from build123d import *

# Parameters (mm, degrees)
F0_W      = 133.35
F0_H      = 57.15
F0_W_2    = 94.615
F0_H_2    = 4.064
F0_W_3    = 10.16
F0_H_3    = 42.545
F1_DEPTH  = 3.81
F2_W      = 5.6896
F2_H      = 39.37
F3_DEPTH  = 31.75
F4_R      = 5.08
F5_R      = 10.287
F6_DEPTH  = 25.4
F7_R      = 2.0701
F8_DEPTH  = 3.811
F9_R      = 5.08
F10_R     = 1.27
F11_R     = 12.7
F11_R_2   = 10.287
F12_DEPTH = 4.6736
F13_DEPTH = 15.494
F14_R     = 2.54
F15_DEPTH = 5.08
F16_R     = 2.54
F17_DEPTH = 25.4
F18_R     = 2.54
F19_DEPTH = 25.4
F20_R     = 2.54
F21_DEPTH = 25.4
F22_R     = 5.07999


# Not quite as in the source:
# - a fillet or chamfer is up to 0.001 mm smaller than in the source, because OpenCascade refuses the exact size


with BuildPart() as f1:
    # F0 (on Top) → F1 (new body)
    with BuildSketch(Plane.XY):
        Rectangle(F0_W, F0_H)
        Polygon((57.4675, -21.2725), (57.4675, -25.3365), (47.3075, -25.3365), (-47.3075, -25.3365), (-57.4675, -25.3365), (-57.4675, -21.2725), (-57.4675, 21.2725), (-57.4675, 25.3365), (-47.3075, 25.3365), (47.3075, 25.3365), (57.4675, 25.3365), (57.4675, 21.2725), align=None, mode=Mode.SUBTRACT)
        with Locations((0, 23.3045)):
            Rectangle(F0_W_2, F0_H_2)
        with Locations((-52.3875, 0)):
            Rectangle(F0_W_3, F0_H_3)
        with Locations((-52.3875, -23.3045)):
            Rectangle(F0_W_3, F0_H_2)
        with Locations((0, -23.3045)):
            Rectangle(F0_W_2, F0_H_2)
        Rectangle(F0_W_2, F0_H_3)
        with Locations((52.3875, 0)):
            Rectangle(F0_W_3, F0_H_3)
        with Locations((52.3875, -23.3045)):
            Rectangle(F0_W_3, F0_H_2)
        with Locations((52.3875, 23.3045)):
            Rectangle(F0_W_3, F0_H_2)
        with Locations((-52.3875, 23.3045)):
            Rectangle(F0_W_3, F0_H_2)
    extrude(amount=F1_DEPTH)

    # F2 (on face) → F3 (join)
    with BuildSketch(Plane.XY.offset(3.81)):
        with Locations((-63.8302, 0.0610498762)):
            Rectangle(F2_W, F2_H)
    extrude(amount=F3_DEPTH)

    # F4
    f4_edges = [f1.edges().sort_by_distance(p)[0] for p in [
        (-63.8302, 19.74605, 35.56),
        (-63.8302, -19.62395, 35.56),
    ]]
    fillet(f4_edges, radius=F4_R)

    # F5 (on face) → F6 (cut)
    with BuildSketch(Plane(origin=(-66.675, 0, 0), x_dir=(0, -1, 0), z_dir=(-1, 0, 0))):
        with Locations((0, 17.145)):
            Circle(F5_R)
    extrude(amount=-F6_DEPTH, mode=Mode.SUBTRACT)

    # F7 (on face) → F8 (cut, through all)
    with BuildSketch(Plane.XY.offset(3.81)):
        with Locations((-62.5474974513, 24.164236586)):
            Circle(F7_R)
        with Locations((62.3570047319, 24.7649991388)):
            Circle(F7_R)
        with BuildLine():
            ThreePointArc((64.4271047319, -24.7650008612), (64.1570098525, -23.7426038856), (63.4172061032, -22.987))
            Line((63.4172061032, -22.987), (61.2968033606, -22.987))
            ThreePointArc((61.2968033606, -22.987), (61.3346077563, -26.5650059818), (64.4271047319, -24.7650008612))
        make_face()
        with BuildLine():
            Line((61.2968033606, -22.987), (63.4172061032, -22.987))
            ThreePointArc((63.4172061032, -22.987), (62.3570047319, -22.6949008612), (61.2968033606, -22.987))
        make_face()
        with Locations((-62.5474974513, -24.7649997473)):
            Circle(F7_R)
    extrude(amount=-F8_DEPTH, mode=Mode.SUBTRACT)

    # F9
    f9_edges = [f1.edges().sort_by_distance(p)[0] for p in [
        (66.675, 28.575, 1.905),
        (-66.675, 28.575, 1.905),
        (-66.675, -28.575, 1.905),
        (66.675, -28.575, 1.905),
    ]]
    fillet(f9_edges, radius=F9_R)

    # F10
    f10_edges = [f1.edges().sort_by_distance(p)[0] for p in [
        (-66.675, 0.06105, 35.56),
    ]]
    fillet(f10_edges, radius=F10_R)

    # F11 (on face) → F12 (cut)
    with BuildSketch(Plane.YZ.offset(-60.9854)):
        with Locations((0, 17.145)):
            Circle(F11_R)
        with Locations((0, 17.145)):
            Circle(F11_R_2, mode=Mode.SUBTRACT)
    extrude(amount=-F12_DEPTH, mode=Mode.SUBTRACT)

    # F0 (on Top) → F13 (join)
    with BuildSketch(Plane.XY):
        with Locations((52.3875, 23.3045)):
            Rectangle(F0_W_3, F0_H_2)
        with Locations((52.3875, -23.3045)):
            Rectangle(F0_W_3, F0_H_2)
        with Locations((-52.3875, 23.3045)):
            Rectangle(F0_W_3, F0_H_2)
        with Locations((-52.3875, -23.3045)):
            Rectangle(F0_W_3, F0_H_2)
    extrude(amount=F13_DEPTH)

    # F14 (on face) → F15 (cut)
    with BuildSketch(Plane(origin=(0, 25.3365, 0), x_dir=(-1, 0, 0), z_dir=(0, 1, 0))):
        with Locations((52.3874983191, 10.1600000635)):
            Circle(F14_R)
    extrude(amount=-F15_DEPTH, mode=Mode.SUBTRACT)

    # F16 (on face) → F17 (cut)
    with BuildSketch(Plane.XZ.offset(25.3365)):
        with Locations((52.3875, 10.16)):
            Circle(F16_R)
    extrude(amount=-F17_DEPTH, mode=Mode.SUBTRACT)

    # F18 (on face) → F19 (cut)
    with BuildSketch(Plane.XZ.offset(-21.2725)):
        with Locations((52.3875, 10.16)):
            Circle(F18_R)
    extrude(amount=-F19_DEPTH, mode=Mode.SUBTRACT)

    # F20 (on face) → F21 (cut)
    with BuildSketch(Plane.XZ.offset(25.3365)):
        with Locations((-52.3875, 10.16)):
            Circle(F20_R)
    extrude(amount=-F21_DEPTH, mode=Mode.SUBTRACT)

    # F22 (radius 5.08 in the source; OpenCascade refuses exactly that, so slightly less here)
    f22_edges = [f1.edges().sort_by_distance(p)[0] for p in [
        (-47.3075, -23.3045, 15.494),
        (-57.4675, -23.3045, 15.494),
        (-57.4675, 23.3045, 15.494),
        (-47.3075, 23.3045, 15.494),
        (47.3075, 23.3045, 15.494),
        (47.3075, -23.3045, 15.494),
        (57.4675, -23.3045, 15.494),
        (57.4675, 23.3045, 15.494),
    ]]
    fillet(f22_edges, radius=F22_R)


solid = f1.part
The listing builds one solid part. Answer for the finished solid, in the listing's coordinates (mm). A direction names the side the tool comes from. Round coordinates to 2 decimals unless told otherwise and drop trailing zeros. Write each loop counter-clockwise with the first axis right and the second up, starting at its lowest first coordinate (ties: lowest second). Pieces come first, ordered by that corner, then holes. Notation, with made-up numbers: (2.5, -29) - (21.5, -29) arc R22 ccw to (21.5, -10) - close; hole circle Ø5 at (48.5, 42.5). An arc over 180 degrees is marked (long way). Use a Markdown table: item, result. Add a question column.
1. The part is cut by section C-C (y = -6). Write down the section's boundary in (x, z) (3 decimals), and give its area (3 significant figures).
2. For a pull along Z with two mould halves and no side action, classify faces 1 (the face through (-63.16, -18.18, 34.03)), 2 (the face through (52, 21.272, 7)), 3 (the face through (-65.659, 4.644, 7.797)) as +Z half, -Z half, draft (parallel to the pull), parting line (faces both ways), or undercut.
3. The part is cut by section D-D (z = 25). Write down the section's boundary in (x, y) (3 decimals), and give its area (3 significant figures).
4. The part is cut by section A-A (y = 0). Write down the section's boundary in (x, z) (3 decimals), and give its area (3 significant figures).
5. Flat-ended cylindrical pins translate along their axes: P1, Ø4, axis at x = -52.39, z = 10.16, coming from the -Y side; P2, Ø17, axis at x = -15, y = -3, coming from the +Z side; P3, Ø5, axis at y = 22, z = 31.5, coming from the -X side; P4, Ø3, axis at x = 54.5, z = 12, coming from the -Y side. Find the tip coordinate at first contact, or state that the pin passes through.
6. The part is cut by section B-B (z = 19). Write down the section's boundary in (x, y) (3 decimals), and give its area (3 significant figures).
7. Consider line 1 (X direction, y = -24, z = 10); line 2 (X direction, y = 15.5, z = 19) (3 decimals); line 3 (X direction, y = -25, z = 6). Determine where each line is inside the solid, lowest interval first.
8. A tool of negligible diameter and unlimited length cuts with its end or side. For faces 4 (the face through (52, 25.336, 7)), 5 (the face through (57.468, 23, 7)), 6 (the face through (-47.308, 23, 7)), 7 (the face through (52, -21.272, 7)), 8 (the face through (-63, -19.624, 17)), from which of +Z, -Z, +X, -X, +Y, -Y can it reach the whole face along a straight path? Write none if from no direction.
Reported:
| question | item | result |
|---|---|---|
| 1 | outline | (-66.675, 0) - (66.675, 0) - (66.675, 3.81) - (-60.985, 3.81) - (-60.985, 5.952) - (-65.659, 5.952) - (-65.659, 8.789) - (-66.675, 8.789) - close; (-66.675, 25.501) - (-65.659, 25.501) - (-65.659, 28.338) - (-60.985, 28.338) - (-60.985, 35.56) - (-65.405, 35.56) arc R1.27 ccw to (-66.675, 34.29) - close |
| 1 | area | 567 mm^2 |
| 2 | face 1 | +Z half |
| 2 | face 2 | draft |
| 2 | face 3 | undercut |
| 3 | outline | (-66.675, -18.354) arc R1.27 ccw to (-65.405, -19.624) - (-60.985, -19.624) - (-60.985, -9.979) - (-65.659, -9.979) - (-65.659, -6.642) - (-66.675, -6.642) - close; (-66.675, 6.642) - (-65.659, 6.642) - (-65.659, 9.979) - (-60.985, 9.979) - (-60.985, 19.746) - (-65.405, 19.746) arc R1.27 ccw to (-66.675, 18.476) - close |
| 3 | area | 117 mm^2 |
| 4 | outline | (-66.675, 0) - (66.675, 0) - (66.675, 3.81) - (-60.985, 3.81) - (-60.985, 4.445) - (-65.659, 4.445) - (-65.659, 6.858) - (-66.675, 6.858) - close; (-66.675, 27.432) - (-65.659, 27.432) - (-65.659, 29.845) - (-60.985, 29.845) - (-60.985, 35.56) - (-65.405, 35.56) arc R1.27 ccw to (-66.675, 34.29) - close |
| 4 | area | 549 mm^2 |
| 5 | P1 | through |
| 5 | P2 | z = 3.81 |
| 5 | P3 | x = -66.05 |
| 5 | P4 | y = -25.34 |
| 6 | outline | (-66.675, -18.354) arc R1.27 ccw to (-65.405, -19.624) - (-60.985, -19.624) - (-60.985, -12.564) - (-65.659, -12.564) - (-65.659, -10.118) - (-66.675, -10.118) - close; (-66.675, 10.118) - (-65.659, 10.118) - (-65.659, 12.564) - (-60.985, 12.564) - (-60.985, 19.746) - (-65.405, 19.746) arc R1.27 ccw to (-66.675, 18.476) - close |
| 6 | area | 85.3 mm^2 |
| 7 | line 1 | -57.47 to -54.92, -49.85 to -47.31, 47.31 to 49.85, 54.92 to 57.47 |
| 7 | line 2 | -66.675 to -60.985 |
| 7 | line 3 | -57.47 to -47.31, 47.31 to 57.47 |
| 8 | face 4 | +Z, +X, -X, +Y |
| 8 | face 5 | +Z, +X, +Y, -Y |
| 8 | face 6 | +Z, +Y, -Y |
| 8 | face 7 | +Z, +X, -X |
| 8 | face 8 | +Z, +X, -X, -Y |
